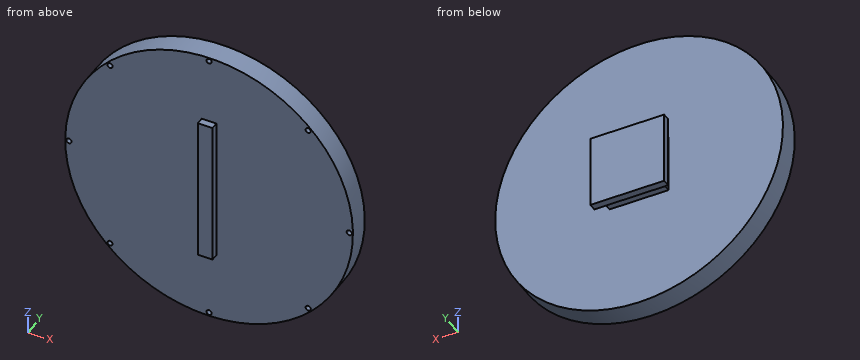
```python
from build123d import *

# Parameters (mm, degrees)
SKETCH1_R           = 49.53
BOSS_EXTRUDE1_DEPTH = 7.62
SKETCH2_R           = 0.889
CUT_EXTRUDE1_DEPTH  = 2.54
CIRPATTERN1_COUNT   = 8
SKETCH4_W           = 5.0546
SKETCH4_H           = 50.546
BOSS_EXTRUDE3_DEPTH = 2.54
SKETCH5_W           = 20.32
SKETCH5_H           = 20.32
BOSS_EXTRUDE4_DEPTH = 5.08
SKETCH6_W           = 25.4
SKETCH6_H           = 25.4
BOSS_EXTRUDE5_DEPTH = 2.54


with BuildPart() as part:
    # Sketch1 → Boss-Extrude1 (new body)
    with BuildSketch(Plane(origin=(0, 0, 0), x_dir=(1, 0, 0), z_dir=(0, 1, 0))):
        with Locations(Location((0, 0, 0), (0, 0, 90))):
            Circle(SKETCH1_R)
    extrude(amount=BOSS_EXTRUDE1_DEPTH)

    # Sketch2 → Cut-Extrude1 (cut)
    with BuildSketch(Plane.XZ):
        with Locations(Location((-48.26, 0, 0), (0, 0, 270))):
            Circle(SKETCH2_R)
    cut_extrude1 = extrude(amount=-CUT_EXTRUDE1_DEPTH, mode=Mode.SUBTRACT)

    # CirPattern1: Cut-Extrude1 ×8 about axis
    cirpattern1_axis = Axis((0, 0, 0), (0, 1, 0))
    for i in range(1, CIRPATTERN1_COUNT):
        add(cut_extrude1.rotate(cirpattern1_axis, i * 360 / CIRPATTERN1_COUNT), mode=Mode.SUBTRACT)

    # Sketch4 → Boss-Extrude3 (add)
    with BuildSketch(Plane.XZ):
        Rectangle(SKETCH4_W, SKETCH4_H)
    extrude(amount=BOSS_EXTRUDE3_DEPTH)

    # Sketch5 → Boss-Extrude4 (add)
    with BuildSketch(Plane(origin=(0, 7.62, 0), x_dir=(1, 0, 0), z_dir=(0, 1, 0))):
        Rectangle(SKETCH5_W, SKETCH5_H)
    extrude(amount=BOSS_EXTRUDE4_DEPTH)

    # Sketch6 → Boss-Extrude5 (add)
    with BuildSketch(Plane(origin=(0, 12.7, 0), x_dir=(1, 0, 0), z_dir=(0, 1, 0))):
        Rectangle(SKETCH6_W, SKETCH6_H)
    extrude(amount=BOSS_EXTRUDE5_DEPTH)


solid = part.part
```
Can you work these out from the model? Positions are in its coordinate system, mm. Coordinates: 2 decimals unless noted, no trailing zeros. Order: outer loops, then holes, each group sorted by start corner. A loop starts at its lowest first (then second) coordinate and runs counter-clockwise, first axis right, second up. Notation, with made-up numbers: (13, 39) - (67, 39) arc R23 ccw to (67, 67) - close; hole circle Ø6 at (49, -36.5). An arc over 180 degrees is marked (long way). Answer in a Markdown table with one row per item.
1. Suppose I cut it at B-B (y = 9). Please give me the cut outline in (x, z), and give its area (3 significant figures).
Reply:
| item | result |
|---|---|
| outline | (-10.16, -10.16) - (10.16, -10.16) - (10.16, 10.16) - (-10.16, 10.16) - close |
| area | 413 mm^2 |
2. Suppose I cut it at C-C (x = -4). Please give me the cut outline in (y, z), and give its area (3 significant figures).
Reply:
| item | result |
|---|---|
| outline | (0, -49.37) - (7.62, -49.37) - (7.62, -10.16) - (12.7, -10.16) - (12.7, -12.7) - (15.24, -12.7) - (15.24, 12.7) - (12.7, 12.7) - (12.7, 10.16) - (7.62, 10.16) - (7.62, 49.37) - (0, 49.37) - close |
| area | 920 mm^2 |
3. Suppose I cut it at A-A (z = 14). Please give me the cut outline in (x, y).
Reply:
| item | result |
|---|---|
| outline | (-47.51, 0) - (-2.53, 0) - (-2.53, -2.54) - (2.53, -2.54) - (2.53, 0) - (47.51, 0) - (47.51, 7.62) - (-47.51, 7.62) - close |
4. If I drill on line 1 along X through (y, z) = (1.65, 0); line 2 along Y through (x, z) = (30.5, 26); line 3 along Z through (x, y) = (10, 11.5), over which ranges is the centre line in solid material (lowest first)?
Reply:
| item | result |
|---|---|
| line 1 | x = -49.53 to -49.15, -47.37 to 47.37, 49.15 to 49.53 |
| line 2 | y = 0 to 7.62 |
| line 3 | z = -10.16 to 10.16 |
5. For pin 1 (5.5 mm diameter, centred on y = 11.5, z = -4, fed in from -X); pin 2 (0.5 mm diameter, centred on x = -48, z = 0, fed in from -Y); pin 3 (2 mm diameter, centred on x = 48.26, z = 0, fed in from -Y), each with a flat end and sliding along its axis, tell me the tip position at first contact or that it passes through.
Reply:
| item | result |
|---|---|
| pin 1 | stops at x = -12.7 |
| pin 2 | stops at y = 2.54 |
| pin 3 | stops at y = 0 |
6. Suppose I cut it at D-D (x = -43). Please give me the cut outline in (y, z).
Reply:
| item | result |
|---|---|
| outline | (0, -24.58) - (7.62, -24.58) - (7.62, 24.58) - (0, 24.58) - close |
